For this review, take the finished solid that the model builds, in its own axes (mm). A direction names the side the tool comes from. Give positions to 0.01 mm unless a question says otherwise; leave off trailing zeros. Loops run counter-clockwise (first coordinate to the right, second up) from the corner with the lowest first, then second, coordinate; pieces in that order, holes last. Notation, with made-up numbers: (-25.75, -31) - (24.25, -31) arc R8 cw to (24.25, -27) - close; hole circle Ø4 at (-11.5, 60). An arc over 180 degrees is marked (long way). Put each result on its own line as item: value. Start each with the question number.
Autodesk Inventor part; units mm, degrees
ref_plane "Start plane" through (0, 0, -10) normal (0, 0, 1) x (1, 0, 0)
ref_plane "End plane" through (0, 0, 160) normal (0, 0, 1) x (1, 0, 0)
ref_plane "Work Plane11" through (-6, 4, -10) normal (0.7071, 0, -0.7071) x (-0.7071, 0, -0.7071)
ref_plane "Start plane" through (0, 0, -10) normal (0, 0, 1) x (1, 0, 0)
ref_plane "End plane" through (0, 0, 160) normal (0, 0, 1) x (1, 0, 0)
sketch "Sketch" plane through (0, 0, 0) normal (0, 0, 1) x (1, 0, 0)
  line L0 (-3, 0.5) -> (-3, 12)
  line L1 (-6, 14) -> (-5, 14)
  line L2 (-6, -6) -> (-6, 14)
  line L3 (-6, -6) -> (14, -6)
  line L4 (14, -5) -> (14, -6)
  line L5 (0.5, -3) -> (12, -3)
  arc A0 (-3, 0.5) -> (0.5, -3) centre (0.5, 0.5) ccw
  arc A1 (-3, 12) -> (-5, 14) centre (-5, 12) ccw
  arc A2 (14, -5) -> (12, -3) centre (12, -5) ccw
  line L6 (0, 18.4971) -> (0, -10.0828) construction
  line L7 (-10.0828, 0) -> (18.4971, 0) construction
  point P0 (-3, -3)
  point P1 (-3, 14)
  point P2 (14, -3)
  dimension "d4" = 20
  dimension "d6" = 20
  dimension "d8" = 3
  dimension "d10" = 3
  dimension "d17" = 3.5
  dimension "d18" = 2
  dimension "d19" = 6
  dimension "d20" = 6
extrude "Body" add sketch "Sketch" along normal up to surface (170 mm away) from surface at -10
sketch "Sketch3" plane through (0, 0, 0) normal (0, 0, 1) x (1, 0, 0)
  line L0 (0, 0) -> (10, 0)
ref_plane "Work Plane10" through (0, 0, 0) normal (0, -1, 0) x (1, 0, 0)
sketch "Sketch4" plane through (0, 0, 0) normal (0, -1, 0) x (1, 0, 0)
  line L0 (-2, -10) -> (12, -10)
  line L1 (-2, 160) -> (12, 160)
  dimension "d24" = 170
ref_plane "Work Plane11" through (-6, 4, -10) normal (0.7071, 0, -0.7071) x (-0.7071, 0, -0.7071)
split "Split1" plane through (-6, 4, -10) removes the side toward (0.7071, 0, -0.7071)
ref_plane "Work Plane12" through (-6, 4, 160) normal (0.7071, 0, 0.7071) x (0.7071, 0, -0.7071)
split "Split2" plane through (-6, 4, 160) removes the side toward (0.7071, 0, 0.7071)
equation "\"d4\" = b"
equation "\"d6\" = b"
equation "\"d17\" = R"
equation "\"d18\" = R1"
equation "\"d19\" = ex"
equation "\"d20\" = d19"
equation "\"d11\" = G_L"
equation "\"b\" = 20"
equation "\"ParT\" = 3"
equation "\"R\" = 3.5"
equation "\"R1\" = 2"
equation "\"G_L\" = d24"
equation "\"ex\" = 6"
equation "\"G_OFFSET_START\" = 10"
equation "\"G_OFFSET_END\" = 10"
equation "\"d21\" = -G_OFFSET_START"
equation "\"d22\" = G_OFFSET_END + B_L"
equation "\"B_L\" = 150"
properties part number "ISO 657-1 - L20x20x3-170" material "Stainless Steel"
1) Take a section at D-D on y = 7.25. State the section outline as (x, z) points, and give its area (3 significant figures).
2) Wall thickness on probe 1 along Y at (x, z) = (12, 126); probe 2 along Y at (x, z) = (-2.5, 149.5): over which ranges is each line inside the solid? List them lowest first.
3) Take a section at A-A on z = 85. State the section outline as (x, y) points.
4) Insertion check: P1, Ø4, axis at x = 0.5, z = 73, coming from the +Y side; P2, Ø6, axis at x = 2, y = -1.5, coming from the -Z side; P3, Ø9, axis at y = 6, z = 57.5, coming from the +X side. Each pin has a flat end and moves straight along its axis. Give the tip position at first contact, or say it passes through.
5) Machinability: for faces 1 (the flat face through (-6, 4, 74)), 2 (the flat face through (6, -3, 74)), which of the approach directions +Z, -Z, +X, -X, +Y, -Y give a long, thin tool a straight path to every point of the face, cutting with its end or side? Answer none if there is none.
6) Take a section at C-C on z = 145. State the section outline as (x, y) points.
7) Take a section at B-B on x = 4.25. State the section outline as (y, z) points, and give its area (4 significant figures).
Answers follow:
1. outline: (-6, -10) - (-3, -7) - (-3, 157) - (-6, 160) - close
1. area: 501 mm2
2. probe 1: -6 to -3
2. probe 2: -6 to -1.3
3. outline: (-6, -6) - (14, -6) - (14, -5) arc R2 ccw to (12, -3) - (0.5, -3) arc R3.5 cw to (-3, 0.5) - (-3, 12) arc R2 ccw to (-5, 14) - (-6, 14) - close
4. P1: y = -2.37
4. P2: z = -4.71
4. P3: x = -3
5. face 1: +Z, -Z, -X, +Y, -Y
5. face 2: +Z, -Z, +X, +Y
6. outline: (-6, -6) - (9, -6) - (9, -3) - (0.5, -3) arc R3.5 cw to (-3, 0.5) - (-3, 12) arc R2 ccw to (-5, 14) - (-6, 14) - close
7. outline: (-6, 0.25) - (-3, 0.25) - (-3, 149.75) - (-6, 149.75) - close
7. area: 448.5 mm2
